Geometry: see drawing. Coordinates: mm, zero at the bounding-box minimum. Give positions to 0.01 mm unless a question says otherwise; leave off trailing zeros. Write each loop counter-clockwise with the first axis right and the second up, starting at its lowest first coordinate (ties: lowest second). Pieces come first, ordered by that corner, then holes. Notation, with made-up numbers: M -30,25.5 L 20,25.5 A20 ccw 20,44.5 Z; hole C -1,-14 d1. An arc over 180 degrees is marked long. Use CSV: the item, a comma, the result in double quotes. Start each with the question number.
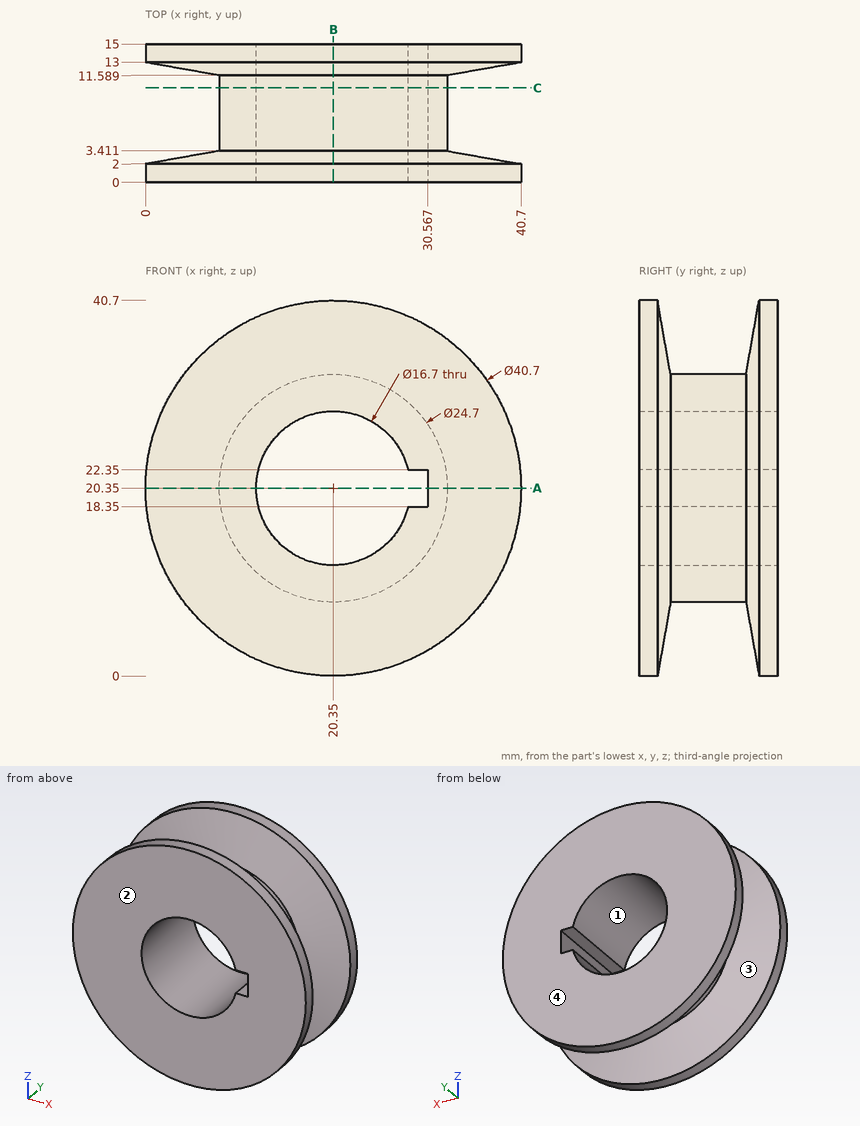
1. Line query: probe 1 along Z at (x, y) = (20.35, 5); probe 2 along Z at (x, y) = (16, 6.5); probe 3 along Y at (x, z) = (13, 39). Output: solid intervals per line, ascending.
2. Section A-A on z = 20.35. Return loops of the section in (x, y).
3. Section B-B on x = 20.35. Return loops of the section in (y, z).
4. First-contact query: pin 1 (6 mm diameter, centred on y = 7, z = 24, fed in from +X); pin 2 (8 mm diameter, centred on x = 4.5, y = 2.5, fed in from +Z); pin 3 (0.6 mm diameter, centred on x = 29.5, y = 9, fed in from -Z) (1 decimal); pin 4 (10 mm diameter, centred on x = 20.35, z = 20.35, fed in from +Y). Flat tips, straight axial feed; report the tip coordinate or a pass-through.
5. Pull-direction query (Y, two-part tool) for the marked faces 1, 2, 3 and 4; classes: released by +Y, released by -Y, zero draft, split by the parting line, or undercut.
6. Section C-C on y = 10.25. Return loops of the section in (x, z), then the cut area to 3 significant figures.
Resolved:
1,probe 1,"z = 8 to 12, 28.7 to 32.7"
1,probe 2,"z = 8.79 to 13.22, 27.48 to 31.91"
1,probe 3,"y = 0 to 2.05, 12.95 to 15"
2,outline,"M 0,0 L 12,0 L 12,15 L 0,15 L 0,13 L 8,11.59 L 8,3.41 L 0,2 Z; M 30.57,0 L 40.7,0 L 40.7,2 L 32.7,3.41 L 32.7,11.59 L 40.7,13 L 40.7,15 L 30.57,15 Z"
3,outline,"M 0,0 L 2,0 L 3.41,8 L 11.59,8 L 13,0 L 15,0 L 15,12 L 0,12 Z; M 0,28.7 L 15,28.7 L 15,40.7 L 13,40.7 L 11.59,32.7 L 3.41,32.7 L 2,40.7 L 0,40.7 Z"
4,pin 1,"stops at x = 32.68"
4,pin 2,"stops at z = 36.87"
4,pin 3,"stops at z = 11.7"
4,pin 4,"passes through"
5,face 1,"zero draft"
5,face 2,"released by -Y"
5,face 3,"undercut"
5,face 4,"released by +Y"
6,outline,"C 20.35,20.35 d24.7; hole M 28.46,18.35 L 30.57,18.35 L 30.57,22.35 L 28.46,22.35 A8.35 ccw long Z"
6,area,"252 mm2"
